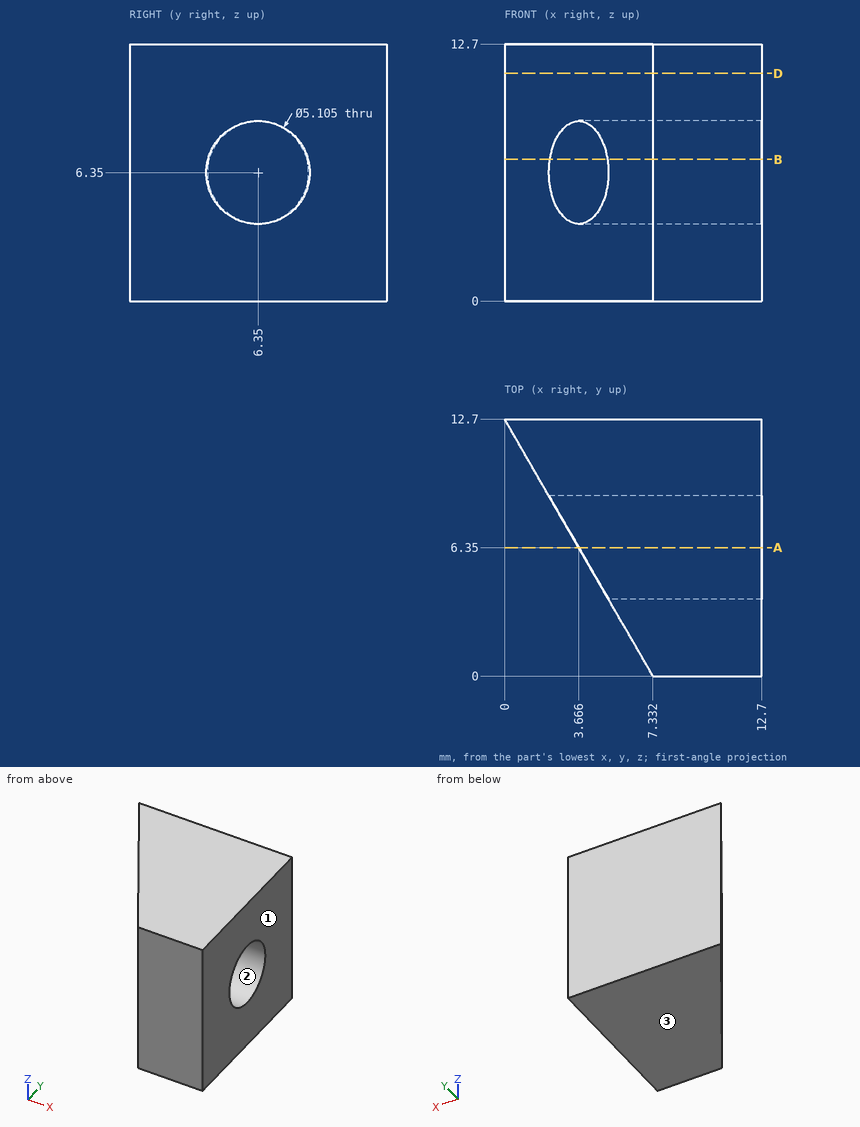
Answer from the drawing. Dimensions are ordinates in mm from the lowest x, y and z of the part. Give positions to 0.01 mm unless a question says otherwise; leave off trailing zeros. Loops run counter-clockwise (first coordinate to the right, second up) from the corner with the lowest first, then second, coordinate; pieces in that order, holes last. Notation, with made-up numbers: (-29.5, 84.25) -> (-11.5, 84.25) arc R26 ccw to (-11.5, 114.25) -> close; hole circle Ø11 at (-4.75, 32). An arc over 180 degrees is marked (long way). Use a Markdown table: item, result.
Q1. Section B-B, the plane z = 7 is taken. Determine the outline of the cut face in (x, y).
Solved:
| item | result |
|---|---|
| outline | (0, 12.7) -> (2.24, 8.82) -> (12.7, 8.82) -> (12.7, 12.7) -> close; (5.09, 3.88) -> (7.33, 0) -> (12.7, 0) -> (12.7, 3.88) -> close |
Q2. Determine the mould class of the marked faces 1, 2 and 3 for opening direction Z: pulls with the +Z half, pulls with the -Z half, needs draft (parallel to the pull), parting line crosses it, or undercut.
Solved:
| item | result |
|---|---|
| face 1 | needs draft |
| face 2 | undercut |
| face 3 | pulls with the -Z half |
Q3. Section D-D, the plane z = 11.25 is taken. Determine the outline of the cut face in (x, y).
Solved:
| item | result |
|---|---|
| outline | (0, 12.7) -> (7.33, 0) -> (12.7, 0) -> (12.7, 12.7) -> close |
Q4. Section A-A, the plane y = 6.35 is taken. Determine the outline of the cut face in (x, z), then the cut area to 3 significant figures.
Solved:
| item | result |
|---|---|
| outline | (3.67, 0) -> (12.7, 0) -> (12.7, 3.8) -> (3.67, 3.8) -> close; (3.67, 8.9) -> (12.7, 8.9) -> (12.7, 12.7) -> (3.67, 12.7) -> close |
| area | 68.6 mm^2 |
Q5. Find the intervals of material crossed by line 1 along Y through (x, z) = (9, 6.35); line 2 along Z through (x, y) = (8.25, 5.5), in increasing order.
Solved:
| item | result |
|---|---|
| line 1 | y = 0 to 3.8, 8.9 to 12.7 |
| line 2 | z = 0 to 3.94, 8.76 to 12.7 |
Q6. Each of these flat-tipped pins is pushed along its axis until it touches: pin 1 (4 mm diameter, centred on y = 9, z = 5.5, fed in from -X); pin 2 (5 mm diameter, centred on y = 7.5, z = 2.5, fed in from -X); pin 3 (3 mm diameter, centred on x = 3.5, z = 6.5, fed in from -Y). Where does it stop, or does it pass through?
Solved:
| item | result |
|---|---|
| pin 1 | stops at x = 0.98 |
| pin 2 | stops at x = 1.56 |
| pin 3 | stops at y = 8.3 |
